Autodesk Inventor part; units mm, degrees
ref_plane "YZ Plane" through (0, 0, 0) normal (1, 0, 0) x (0, 1, 0)
ref_plane "XZ Plane" through (0, 0, 0) normal (0, 1, 0) x (-1, 0, 0)
ref_plane "XY Plane" through (0, 0, 0) normal (0, 0, 1) x (1, 0, 0)
sketch "Sketch1" plane through (0, 0, 0) normal (0, 1, 0) x (-1, 0, 0)
  line L0 (44.45, 44.45) -> (-44.45, 44.45)
  line L1 (-44.45, 44.45) -> (-44.45, -44.45)
  line L2 (-44.45, -44.45) -> (44.45, -44.45)
  line L3 (44.45, -44.45) -> (44.45, 44.45)
  line L4 (44.45, 44.45) -> (-44.45, -44.45) construction
  line L5 (-44.45, 44.45) -> (44.45, -44.45) construction
  point P0 (0, 0)
  dimension "d0" = 88.9
  dimension "d1" = 88.9
extrude "Extrusion1" add sketch "Sketch1" along normal blind 5
sketch "Sketch2" plane through (0, 5, 0) normal (0, 1, 0) x (1, 0, 0)
  circle A0 centre (0, 0) radius 25.4
  dimension "d4" = 50.8
extrude "Extrusion2" add sketch "Sketch2" along normal blind 50
sketch "Sketch3" plane through (0, 5, 0) normal (0, 1, 0) x (1, 0, 0)
  line L0 (44.45, 44.45) -> (-44.45, 44.45)
  line L1 (-44.45, 44.45) -> (-44.45, -44.45)
  line L2 (44.45, -44.45) -> (44.45, 44.45)
  line L3 (-44.45, -44.45) -> (44.45, -44.45)
  point P0 (0, 0)
  point P1 (-34.45, 34.45)
  point P2 (0, 34.45)
  point P3 (34.45, 34.45)
  point P4 (34.45, 0)
  point P5 (34.45, -34.45)
  point P6 (0, -34.45)
  point P7 (-34.45, -34.45)
  point P8 (-34.45, 0)
  dimension "d14" = 10
  dimension "d15" = 10
  dimension "d16" = 10
  dimension "d17" = 0
  dimension "d18" = 10
  dimension "d19" = 10
  dimension "d20" = 10
  dimension "d21" = 0
  dimension "d22" = 10
  dimension "d23" = 10
  dimension "d24" = 10
  dimension "d25" = 0
  dimension "d26" = 10
  dimension "d27" = 10
  dimension "d28" = 10
  dimension "d29" = 0
hole "Hole1" at (-34.45, 5, -34.45) at (0, 5, -34.45) at (34.45, 5, -34.45) at (34.45, 5, 0) at (34.45, 5, 34.45) at (0, 5, 34.45) at (-34.45, 5, 34.45) at (-34.45, 5, 0) direction (0, -1, 0) diameter 4.496 end through all
sketch "Sketch4" plane through (0, 55, 0) normal (0, 1, 0) x (1, 0, 0)
  circle A0 centre (0, 0) radius 21.9
  dimension "d30" = 43.8
extrude "Extrusion3" cut sketch "Sketch4" against normal up to next
fillet "Fillet1" radius 5 4 edges at (-44.45, 2.5, 44.45) (44.45, 2.5, 44.45) (44.45, 2.5, -44.45) (-44.45, 2.5, -44.45)
properties part number "duct_mount"
Check sheet for the modelled part. Datum: model origin and axes. Units: mm. A direction names the side the tool comes from. Round coordinates to 2 decimals unless told otherwise and drop trailing zeros. Write each loop counter-clockwise with the first axis right and the second up, starting at its lowest first coordinate (ties: lowest second). Pieces come first, ordered by that corner, then holes. Notation, with made-up numbers: (-16.75, -14.5) - (42.25, -14.5) arc R28 ccw to (42.25, 11.5) - close; hole circle Ø9 at (-13, 28.25). An arc over 180 degrees is marked (long way). Return JSON: item names as keys, results as strings.
Q1. Cross-section at A-A (x = -34.45). Record the boundary of the cut face in (y, z), then the cut area to 3 significant figures.
Returned:
{"outline": "(0, -44.45) - (5, -44.45) - (5, -36.7) - (0, -36.7) - close; (0, -32.2) - (5, -32.2) - (5, -2.25) - (0, -2.25) - close; (0, 2.25) - (5, 2.25) - (5, 32.2) - (0, 32.2) - close; (0, 36.7) - (5, 36.7) - (5, 44.45) - (0, 44.45) - close", "area": "377 mm²"}
Q2. Depth check by flat-ended pin: P1, Ø5, axis at x = -34.45, z = -34.45, coming from the -Y side; P2, Ø3.5, axis at x = 0, z = -34.45, coming from the +Y side; P3, Ø4, axis at y = 46, z = 6, coming from the +X side; P4, Ø5, axis at x = 34.45, z = -34.45, coming from the +Y side. Enter the tip coordinate at first touch or a pass-through.
Returned:
{"P1": "stops at y = 0", "P2": "passes through", "P3": "stops at x = 25.08", "P4": "stops at y = 5"}
Q3. Draft check along X on faces 1 (the flat face through (-1, 2, 44.45)), 2 (the cylindrical face through (-36.346, 2.465, -33.241)), 3 (the cylindrical face through (42.95, 2.54, 43.02)). Enter one of: released by +X, released by -X, zero draft, split by the parting line, or undercut.
Returned:
{"face 1": "zero draft", "face 2": "undercut", "face 3": "released by +X"}
Q4. Cross-section at B-B (z = -34.45). Record the boundary of the cut face in (x, y), then the cut area to 3 significant figures.
Returned:
{"outline": "(-44.45, 0) - (-36.7, 0) - (-36.7, 5) - (-44.45, 5) - close; (-32.2, 0) - (-2.25, 0) - (-2.25, 5) - (-32.2, 5) - close; (2.25, 0) - (32.2, 0) - (32.2, 5) - (2.25, 5) - close; (36.7, 0) - (44.45, 0) - (44.45, 5) - (36.7, 5) - close", "area": "377 mm²"}
Q5. Scan lines: L1, parallel to X at y = 2.75, z = 0; L2, parallel to Z at x = -34.45, y = 1.5; L3, parallel to X at y = 2, z = 34. Record each from-to range of solid material in increasing order. Write a range as from..to.
Returned:
{"L1": "x = -44.45..-36.7, -32.2..-21.9, 21.9..32.2, 36.7..44.45", "L2": "z = -44.45..-36.7, -32.2..-2.25, 2.25..32.2, 36.7..44.45", "L3": "x = -44.45..-36.65, -32.25..-2.2, 2.2..32.25, 36.65..44.45"}
Q6. Cross-section at D-D (y = 21). Record the boundary of the cut face in (x, z), then the cut area to 3 significant figures.
Returned:
{"outline": "circle Ø50.8 at (0, 0); hole circle Ø43.8 at (0, 0)", "area": "520 mm²"}
Q7. Cross-section at C-C (z = 19). Record the boundary of the cut face in (x, y).
Returned:
{"outline": "(-44.45, 0) - (-10.89, 0) - (-10.89, 55) - (-16.86, 55) - (-16.86, 5) - (-44.45, 5) - close; (10.89, 0) - (44.45, 0) - (44.45, 5) - (16.86, 5) - (16.86, 55) - (10.89, 55) - close"}
Q8. Access from +Z, -Z, +X, -X, +Y, -Y to the whole of each face (thin tool, end or side, straight path). Record for faces 4 (the cylindrical face through (-17.4, 27.9, 13.3)), 5 (the flat face through (-19, 5, 20)).
Returned:
{"face 4": "+Y, -Y", "face 5": "+Y"}
